Verification items for the finished model (mm, model axes). A direction names the side the tool comes from. Round coordinates to 2 decimals unless told otherwise and drop trailing zeros. Write each loop counter-clockwise with the first axis right and the second up, starting at its lowest first coordinate (ties: lowest second). Pieces come first, ordered by that corner, then holes. Notation, with made-up numbers: M 75,77.25 L 118,77.25 A6 cw 118,83.25 Z; hole C 58,-4.5 d8. An arc over 180 degrees is marked long. One line per item, written item: value. Start each with the question number.
Item 1: Gauge pin test, flat ends, axial feed: pin 1 (5 mm diameter, centred on x = 1.5, z = -23, fed in from +Y); pin 2 (4 mm diameter, centred on x = 4, y = 12, fed in from -Z); pin 3 (5 mm diameter, centred on x = -1.5, y = 16, fed in from +Z); pin 4 (14.5 mm diameter, centred on y = 25, z = 0, fed in from +X). Record the tip position at first contact, or that the pin passes through.
Item 2: Draft check along Z on faces 1 (the face through (-5, 15, 0)), 2 (the face through (0, 3, -27)), 3 (the face through (-0.07, 29.868, 6.349)). Enter one of: +Z half, -Z half, draft (parallel to the pull), parting line (faces both ways), or undercut.
Item 3: Section check A-A, the plane y = 25. Record the cut outline in (x, z), then the cut area to 3 significant figures.
Item 4: Tool access check on faces 4 (the face through (-0.676, 3.042, -23.146)), 5 (the face through (1.438, 36.18, 0.748)), 6 (the face through (0, 3, 27)), 7 (the face through (0, 23, 15)), 8 (the face through (-2.3, 6, -19.8)). Record the directions out of +Z, -Z, +X, -X, +Y, -Y that give a thin tool (end or side, any length) a straight path to the whole face; none if there is none.
Item 5: Section check C-C, the plane x = 0. Record the cut outline in (y, z).
Item 6: Section check B-B, the plane z = 21. Record the cut outline in (x, y).
Item 7: Thickness scan on probe 1 along Z at (x, y) = (0, 2.8); probe 2 along Z at (x, y) = (0, 35); probe 3 along Z at (x, y) = (-3, 25). Record the ranges inside material, lowest first. Write a range as from..to.
Item 8: Section check D-D, the plane z = 0. Record the cut outline in (x, y).
Autodesk Inventor part; units mm, degrees
ref_plane "b_s_XY" through (0, 33, 0) normal (0, 1, 0) x (1, 0, 0)
ref_plane "b_s_YZ" through (0, 33, 0) normal (1, 0, 0) x (0, 0, -1)
ref_plane "b_s_ZX" through (0, 33, 0) normal (0, 0, -1) x (0, 1, 0)
sketch "Sketch_1" plane through (0, 0, 0) normal (1, 0, 0) x (0, 1, 0)
  line L0 (6, 27) -> (0, 27)
  line L1 (0, 27) -> (0, -27)
  line L2 (0, -27) -> (6, -27)
  line L3 (6, -27) -> (6, -15)
  line L4 (6, -15) -> (40, -15)
  line L5 (40, -15) -> (40, 15)
  line L6 (40, 15) -> (6, 15)
  line L7 (6, 15) -> (6, 27)
extrude "Extrusion1" add sketch "Sketch_1" along normal mid plane 10
sketch "Sketch2" plane through (-5, 40, 15) normal (0, 1, 0) x (1, 0, 0)
  point P0 (5, 15)
hole "Hole1" at (0, 40, 0) direction (0, -1, 0) diameter 3.242 depth 14.0641 tip angle 120 countersink diameter 4 countersink angle 90
sketch "Sketch3" plane through (-5, 0, -27) normal (0, -1, 0) x (1, 0, 0)
  point P0 (5, 6)
hole "Hole2" at (0, 0, -21) direction (0, 1, 0) diameter 4.5 depth 6
pattern_linear "Rectangular Pattern1" count 2 spacing 42 along (0, 0, 1) of "Hole2"
sketch "Sketch4" plane through (5, 0, 0) normal (1, 0, 0) x (0, 0, -1)
  point P0 (0, 25)
hole "Hole3" at (5, 25, 0) direction (-1, 0, 0) diameter 16 depth 10
ref_plane "b_s_XY" through (0, 33, 0) normal (0, 1, 0) x (1, 0, 0)
ref_plane "b_s_YZ" through (0, 33, 0) normal (1, 0, 0) x (0, 0, -1)
ref_plane "b_s_ZX" through (0, 33, 0) normal (0, 0, -1) x (0, 1, 0)
properties part number "SHTA16-25_b"
Response values:
1. pin 1: stops at y = 6
1. pin 2: stops at z = -15
1. pin 3: stops at z = 15
1. pin 4: passes through
2. face 1: draft
2. face 2: -Z half
2. face 3: undercut
3. outline: M -5,-15 L 5,-15 L 5,-8 L -5,-8 Z; M -5,8 L 5,8 L 5,15 L -5,15 Z
3. area: 140 mm2
4. face 4: +Y, -Y
4. face 5: +Y
4. face 6: +Z, +X, -X, +Y, -Y
4. face 7: +Z, +X, -X, +Y
4. face 8: -Z, +X, -X, +Y
5. outline: M 0,-27 L 6,-27 L 6,-23.25 L 0,-23.25 Z; M 0,-18.75 L 6,-18.75 L 6,-15 L 40,-15 L 40,-2 L 39.62,-1.62 L 32.83,-1.62 A8 cw long 32.83,1.62 L 39.62,1.62 L 40,2 L 40,15 L 6,15 L 6,18.75 L 0,18.75 Z; M 0,23.25 L 6,23.25 L 6,27 L 0,27 Z
6. outline: M -5,0 L -2.25,0 L -2.25,6 L -5,6 Z; M 2.25,0 L 5,0 L 5,6 L 2.25,6 Z
7. probe 1: z = -27..-23.25, -18.75..18.75, 23.25..27
7. probe 2: z = -15..-1.62, 1.62..15
7. probe 3: z = -15..-8, 8..15
8. outline: M -5,0 L 5,0 L 5,17 L -5,17 Z; M -5,33 L -1.62,33 L -1.62,39.62 L -2,40 L -5,40 Z; M 1.62,33 L 5,33 L 5,40 L 2,40 L 1.62,39.62 Z
